Part model, mm, in its own coordinate system. Face numbers are marked on the shaded views. Give positions to 0.01 mm unless a question says otherwise; leave off trailing zeros. Write each loop counter-clockwise with the first axis right and the second up, starting at its lowest first coordinate (ties: lowest second). Pieces come first, ordered by that corner, then holes. Notation, with made-up numbers: M 14.25,25.5 L 55.25,25.5 A19 cw 55.25,47.5 Z; hole C 13,-22.75 d7. An arc over 180 degrees is marked long. Use a Markdown table: item, result. Add a question column.
from build123d import *

# Parameters (mm, degrees)
SKETCH1_R                  = 2.4638
BASE_FLANGE1_DEPTH         = 3.175
SKETCHED_START             = -25.4
SKETCHED_BEND1_DEPTH       = 50.8
SKETCHED_START_2           = -10.2361999
SKETCHED_BEND1_2_DEPTH     = 20.4723998
SKETCHED_START_3           = -22.86
SKETCHED_BEND1_3_DEPTH     = 7.6961999
SKETCHED_START_4           = 15.1638001
SKETCHED_BEND1_4_DEPTH     = 7.6961999
SKETCHED_BEND1_5_DEPTH     = 50.8
SKETCHED_START_5           = -21.302020374
SKETCHED_BEND1_6_OUTLINE_R = 2.4638
SKETCHED_BEND1_6_DEPTH     = 4.302020374


with BuildPart() as part:
    # Base-Flange1: sheet metal written as solids
    # Sketch1 → Base-Flange1 (new body)
    with BuildSketch(Plane(origin=(0, 0, 0), x_dir=(1, 0, 0), z_dir=(0, 1, 0))):
        with BuildLine():
            Line((-29.5783, 25.4), (-126.842248776, -71.863948776))
            ThreePointArc((-126.842248776, -71.863948776), (-127.392851564, -74.632015918), (-125.046197552, -76.2))
            Line((-125.046197552, -76.2), (-60.38835348, -76.2))
            ThreePointArc((-60.38835348, -76.2), (-59.416337562, -76.006654013), (-58.592302256, -75.456051224))
            Line((-58.592302256, -75.456051224), (-30.322248776, -47.185997744))
            ThreePointArc((-30.322248776, -47.185997744), (-29.771645987, -46.361962438), (-29.5783, -45.38994652))
            Line((-29.5783, -45.38994652), (-29.5783, -25.4))
            Line((-29.5783, -25.4), (27.0383, -25.4))
            ThreePointArc((27.0383, -25.4), (28.834351224, -24.656051224), (29.5783, -22.86))
            Line((29.5783, -22.86), (29.5783, 22.86))
            ThreePointArc((29.5783, 22.86), (28.834351224, 24.656051224), (27.0383, 25.4))
            Line((27.0383, 25.4), (-29.5783, 25.4))
        make_face()
        with Locations(Location((-77.296763274, -58.239487758, 0), (0, 0, 270))):
            Circle(SKETCH1_R, mode=Mode.SUBTRACT)
        with Locations(Location((-59.336251031, -40.278975516, 0), (0, 0, 270))):
            Circle(SKETCH1_R, mode=Mode.SUBTRACT)
        with Locations(Location((4.1783, -12.7, 0), (0, 0, 270))):
            Circle(SKETCH1_R, mode=Mode.SUBTRACT)
        with Locations(Location((4.1783, 12.7, 0), (0, 0, 270))):
            Circle(SKETCH1_R, mode=Mode.SUBTRACT)
    extrude(amount=-BASE_FLANGE1_DEPTH)

    # Sketched Bend1: read off the stored shape, not the designer's step
    # Sketched Bend1 outline → Sketched Bend1 (cut)
    with BuildSketch(Plane.XY.offset(SKETCHED_START)):
        with BuildLine():
            Line((29.5783, 0), (-19.570493847, 0))
            ThreePointArc((-19.570493847, 0), (-20.920192704, -2.278520157), (-23.412112646, -3.175))
            Line((-23.412112646, -3.175), (29.5783, -3.175))
            Line((29.5783, -3.175), (29.5783, 0))
        make_face()
    extrude(amount=SKETCHED_BEND1_DEPTH, mode=Mode.SUBTRACT)

    # Sketched Bend1 2 outline → Sketched Bend1 2 (add)
    with BuildSketch(Plane.XY.offset(SKETCHED_START_2)):
        with BuildLine():
            ThreePointArc((-19.570493847, 0), (-19.508115407, 0.98036242), (-19.691959977, 1.945350875))
            Line((-19.691959977, 1.945350875), (-34.713148559, 48.175815683))
            Line((-34.713148559, 48.175815683), (-37.732752998, 47.194686726))
            Line((-37.732752998, 47.194686726), (-22.711564416, 0.964221918))
            ThreePointArc((-22.711564416, 0.964221918), (-22.816190728, 0.303637383), (-23.412112646, 0))
            Line((-23.412112646, 0), (-19.570493847, 0))
        make_face()
    extrude(amount=SKETCHED_BEND1_2_DEPTH)

    # Sketched Bend1 3 outline → Sketched Bend1 3 (add)
    with BuildSketch(Plane.XY.offset(SKETCHED_START_3)):
        with BuildLine():
            ThreePointArc((-19.570493847, 0), (-19.508115407, 0.98036242), (-19.691959977, 1.945350875))
            Line((-19.691959977, 1.945350875), (-34.713148559, 48.175815683))
            Line((-34.713148559, 48.175815683), (-37.732752998, 47.194686726))
            Line((-37.732752998, 47.194686726), (-22.711564416, 0.964221918))
            ThreePointArc((-22.711564416, 0.964221918), (-22.816190728, 0.303637383), (-23.412112646, 0))
            Line((-23.412112646, 0), (-19.570493847, 0))
        make_face()
    extrude(amount=SKETCHED_BEND1_3_DEPTH)

    # Sketched Bend1 4 outline → Sketched Bend1 4 (add)
    with BuildSketch(Plane.XY.offset(SKETCHED_START_4)):
        with BuildLine():
            ThreePointArc((-19.570493847, 0), (-19.508115407, 0.98036242), (-19.691959977, 1.945350875))
            Line((-19.691959977, 1.945350875), (-34.713148559, 48.175815683))
            Line((-34.713148559, 48.175815683), (-37.732752998, 47.194686726))
            Line((-37.732752998, 47.194686726), (-22.711564416, 0.964221918))
            ThreePointArc((-22.711564416, 0.964221918), (-22.816190728, 0.303637383), (-23.412112646, 0))
            Line((-23.412112646, 0), (-19.570493847, 0))
        make_face()
    extrude(amount=SKETCHED_BEND1_4_DEPTH)

    # Sketched Bend1 5 outline → Sketched Bend1 5 (add)
    with BuildSketch(Plane.XY.offset(SKETCHED_START)):
        with BuildLine():
            ThreePointArc((-19.570493847, 0), (-19.508115407, 0.98036242), (-19.691959977, 1.945350875))
            Line((-19.691959977, 1.945350875), (-34.713148559, 48.175815683))
            Line((-34.713148559, 48.175815683), (-37.732752998, 47.194686726))
            Line((-37.732752998, 47.194686726), (-22.711564416, 0.964221918))
            ThreePointArc((-22.711564416, 0.964221918), (-22.816190728, 0.303637383), (-23.412112646, 0))
            Line((-23.412112646, 0), (-19.570493847, 0))
        make_face()
    extrude(amount=SKETCHED_BEND1_5_DEPTH)

    # Sketched Bend1 6 outline → Sketched Bend1 6 (cut)
    with BuildSketch(Plane(origin=(0, 0, 0), x_dir=(-0.30901699437495117, 0.9510565162951524, 0), z_dir=(0.9510565162951524, 0.3090169943749511, 0)).offset(SKETCHED_START_5)):
        with BuildLine():
            Line((56.544876266, -25.4), (56.544876266, -22.86))
            ThreePointArc((56.544876266, -22.86), (55.80092749, -24.656051224), (54.004876266, -25.4))
            Line((54.004876266, -25.4), (56.544876266, -25.4))
        make_face()
        with BuildLine():
            ThreePointArc((54.004876266, 25.4), (55.80092749, 24.656051224), (56.544876266, 22.86))
            Line((56.544876266, 22.86), (56.544876266, 25.4))
            Line((56.544876266, 25.4), (54.004876266, 25.4))
        make_face()
        with Locations((31.144876266, 12.7)):
            Circle(SKETCHED_BEND1_6_OUTLINE_R)
        with Locations((31.144876266, -12.7)):
            Circle(SKETCHED_BEND1_6_OUTLINE_R)
    extrude(amount=SKETCHED_BEND1_6_DEPTH, mode=Mode.SUBTRACT)


solid = part.part
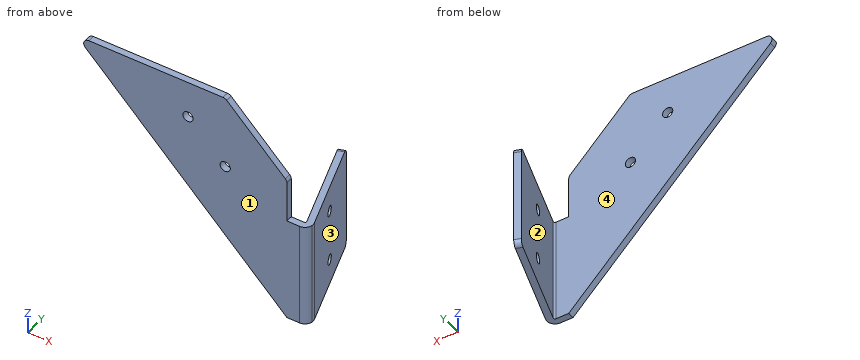
1. Flat gauge pins, fed straight in: pin 1 (5 mm diameter, centred on y = 10, z = -8, fed in from -X); pin 2 (10 mm diameter, centred on x = -101, z = 43.5, fed in from -Y) (3 decimals); pin 3 (5 mm diameter, centred on x = -74, z = 20, fed in from +Y); pin 4 (1 mm diameter, centred on y = -1, z = 34.5, fed in from +X). Where does each tip first touch, or does it go through?
2. Cut at B-B (y = 24). Give the number of separate pieces and of enclosed holes in the cut face, then the cut area to 3 significant figures.
3. Cut at A-A (z = 57.5). Write the cut outline in (x, y) (3 decimals), then the cut area to 3 significant figures.
4. Drill centre lines: probe 1 along Y at (x, z) = (-38, 39.5) (3 decimals); probe 2 along X at (y, z) = (12, 10); probe 3 along X at (y, z) = (33, 9). Where is each one in solid material? Low to high. Write a range as [from, to].
5. Mould opens along Y. For the marked faces 1, 2, 3 and 4 say: released by +Y, released by -Y, zero draft, split by the parting line, or undercut.
6. Cut at D-D (x = -50). Write the cut outline in (y, z) (3 decimals), then the cut area to 3 significant figures.
7. Cut at C-C (z = 40). Write the cut outline in (x, y) (3 decimals), then the cut area to 3 significant figures.
A:
| question | item | result |
|---|---|---|
| 1 | pin 1 | stops at x = -26.46 |
| 1 | pin 2 | stops at y = -3.175 |
| 1 | pin 3 | stops at y = 0 |
| 1 | pin 4 | stops at x = -29.58 |
| 2 | separate pieces | 3 |
| 2 | enclosed holes | 0 |
| 2 | area | 138 mm² |
| 3 | outline | M -112.478,-3.175 L -79.647,-3.175 L -79.647,0 L -112.478,0 Z; M -74.947,-3.175 L -40.636,-3.175 L -40.636,0 L -74.947,0 Z |
| 3 | area | 213 mm² |
| 4 | probe 1 | y = [-3.175, 0] |
| 4 | probe 2 | x = [-26.3, -22.96] |
| 4 | probe 3 | x = [-33.12, -29.78] |
| 5 | face 1 | released by -Y |
| 5 | face 2 | undercut |
| 5 | face 3 | released by +Y |
| 5 | face 4 | undercut |
| 6 | outline | M -3.175,-4.978 L 0,-4.978 L 0,66.864 L -3.175,66.864 Z |
| 6 | area | 228 mm² |
| 7 | outline | M -94.978,-3.175 L -61.784,-3.175 L -61.784,0 L -94.978,0 Z; M -56.888,-3.175 L -29.578,-3.175 L -29.578,0 L -56.888,0 Z |
| 7 | area | 192 mm² |
